Autodesk Inventor part; units mm, degrees
ref_plane "YZ Plane" through (0, 0, 0) normal (1, 0, 0) x (0, 1, 0)
ref_plane "XZ Plane" through (0, 0, 0) normal (0, 1, 0) x (-1, 0, 0)
ref_plane "XY Plane" through (0, 0, 0) normal (0, 0, 1) x (1, 0, 0)
sketch "Sketch1" plane through (0, 0, 0) normal (0, 0, 1) x (1, 0, 0)
  line L0 (-32.5, 20) -> (32.5, 20)
  line L1 (32.5, 20) -> (32.5, -20)
  line L2 (32.5, -20) -> (-32.5, -20)
  line L3 (-32.5, -20) -> (-32.5, 20)
  point P0 (0, 0)
  point P1 (0, 20)
  point P2 (-32.5, 0)
  dimension "d0" = 65
  dimension "d1" = 40
extrude "Extrusion1" add sketch "Sketch1" along normal blind 8
sketch "Sketch5" plane through (0, 0, 0) normal (0, 0, -1) x (-1, 0, 0)
  line L0 (-32.5, 40) -> (0.5, 40)
  line L1 (0.5, 40) -> (0.5, -40)
  line L2 (0.5, -40) -> (-32.5, -40)
  line L3 (-32.5, -40) -> (-32.5, 40)
  line L4 (-32.5, -20) -> (-32.5, 20)
  line L5 (-32.5, 20) -> (32.5, 20)
  line L6 (32.5, -20) -> (-32.5, -20)
  point P0 (0, 0)
  dimension "d22" = 20
  dimension "d23" = 20
  dimension "d24" = 33
extrude "Extrusion5" add sketch "Sketch5" against normal up to surface (8 mm away)
sketch "Sketch6" plane through (0, 0, 0) normal (0, 0, -1) x (-1, 0, 0)
  line L0 (0.5, 40) -> (-32.5, 40)
  line L1 (-32.5, 40) -> (-32.5, -40)
  line L2 (-15, 16.5) -> (16, 16.5) construction
  line L3 (16, 16.5) -> (16, -14.5) construction
  line L4 (16, -14.5) -> (-15, -14.5) construction
  line L5 (-15, -14.5) -> (-15, 16.5) construction
  line L6 (-15, 16.5) -> (16, -14.5) construction
  line L7 (16, 16.5) -> (-15, -14.5) construction
  circle A0 centre (-15, 16.5) radius 1.75
  circle A1 centre (16, 16.5) radius 1.75
  circle A2 centre (16, -14.5) radius 1.75
  circle A3 centre (-15, -14.5) radius 1.75
  circle A4 centre (0.5, 1) radius 8.5
  dimension "d29" = 31
  dimension "d30" = 33
  dimension "d31" = 39
  dimension "d32" = 3.5
  dimension "d33" = 17
extrude "Extrusion6" cut sketch "Sketch6" against normal blind 10
sketch "Sketch7" plane through (0, 0, 0) normal (0, 0, -1) x (-1, 0, 0)
  line L0 (-32.5, 40) -> (-32.5, -40)
  line L1 (0.5, 40) -> (-32.5, 40)
  line L2 (0.5, 20) -> (0.5, 40)
  line L3 (-32.5, -40) -> (0.5, -40)
  point P0 (0, 0)
  point P1 (-24.5, 32)
  point P2 (-7.5, 32)
  point P3 (-24.5, -32)
  point P4 (-7.5, -32)
  dimension "d36" = 8
  dimension "d37" = 8
  dimension "d38" = 8
  dimension "d39" = 17
  dimension "d40" = 8
  dimension "d41" = 64
hole "Hole1" at (24.5, 32, 0) direction (0, 0, 1) diameter 5 end through all
pattern_linear "Rectangular Pattern1" count 2 spacing 64 along (0, -1, 0) count 2 spacing 17 along (-1, 0, 0) of "Hole1"
equation "\"d23\" = d22"
properties part number "0005-10-023 Suport motor x" material "Wood (Maple)"
Geometry check sheet. Reference: the model listing, model coordinates, mm. A direction names the side the tool comes from. Give positions to 0.01 mm unless a question says otherwise; leave off trailing zeros. Order: outer loops, then holes, each group sorted by start corner. A loop starts at its lowest first (then second) coordinate and runs counter-clockwise, first axis right, second up.
1. Section check D-D, the plane x = -3. Enter the section's corners in (y, z), and give its area (3 significant figures).
2. Section check B-B, the plane x = 24.5. Enter the section's corners in (y, z), and give its area (3 significant figures).
3. Section check A-A, the plane y = 32. Enter the section's corners in (x, z).
4. Gauge pin test, flat ends, axial feed: pin 1 Ø4 at (x, z) = (-10, 2.5) entering from -Y; pin 2 Ø3 at (x, y) = (24.5, 32) entering from -Z; pin 3 Ø2.5 at (y, z) = (-28.5, 5) entering from -X; pin 4 Ø4 at (x, z) = (-9.5, 2.5) entering from +Y. Record the tip position at first contact, or that the pin passes through.
5. Release check for a two-part mould opening along Y. For faces 4 (the face through (-16, -20, 4)), 5 (the face through (22, 32, 4)), 6 (the face through (32.5, 1, 4)), 7 (the face through (-15.772, -12.765, 3.944)) record: pulls with the +Y half, pulls with the -Y half, needs draft (parallel to the pull), parting line crosses it, or undercut.
6. Thickness scan on L1, parallel to Y at x = -16, z = 1.75; L2, parallel to X at y = -32, z = 6; L3, parallel to Y at x = 24.5, z = 4.75. Record the ranges inside material, lowest first.
7. Section check C-C, the plane z = 2. Give the number of separate pieces and of enclosed holes in the cut face, and give its area (3 significant figures).
8. Access from +Z, -Z, +X, -X, +Y, -Y to the whole of each face (thin tool, end or side, straight path). Record for faces 1 (the face through (-0.5, 30, 4)), 2 (the face through (-0.5, -30, 4)), 3 (the face through (22, -32, 4)).
Values follow:
1. outline: (-20, 0) - (-7.12, 0) - (-7.12, 8) - (-20, 8) - close; (9.12, 0) - (20, 0) - (20, 8) - (9.12, 8) - close
1. area: 190 mm2
2. outline: (-40, 0) - (-34.5, 0) - (-34.5, 8) - (-40, 8) - close; (-29.5, 0) - (29.5, 0) - (29.5, 8) - (-29.5, 8) - close; (34.5, 0) - (40, 0) - (40, 8) - (34.5, 8) - close
2. area: 560 mm2
3. outline: (-0.5, 0) - (5, 0) - (5, 8) - (-0.5, 8) - close; (10, 0) - (22, 0) - (22, 8) - (10, 8) - close; (27, 0) - (32.5, 0) - (32.5, 8) - (27, 8) - close
4. pin 1: stops at y = -20
4. pin 2: passes through
4. pin 3: stops at x = -0.5
4. pin 4: stops at y = 20
5. face 4: pulls with the -Y half
5. face 5: undercut
5. face 6: needs draft
5. face 7: undercut
6. L1: y = -20 to -16.25, -12.75 to 14.75, 18.25 to 20
6. L2: x = -0.5 to 5, 10 to 22, 27 to 32.5
6. L3: y = -40 to -34.5, -29.5 to 29.5, 34.5 to 40
7. separate pieces: 1
7. enclosed holes: 9
7. area: 3,580 mm2
8. face 1: +Z, -Z, -X, +Y
8. face 2: +Z, -Z, -X, -Y
8. face 3: +Z, -Z
